```python
from build123d import *

# Parameters (mm, degrees)
SKETCH1_R           = 15.875
BOSS_EXTRUDE1_DEPTH = 50.8
SKETCH2_R           = 6.35
BOSS_EXTRUDE2_DEPTH = 6.35
SKETCH3_R           = 1.5875
BOSS_EXTRUDE3_DEPTH = 3.175
SKETCH4_R           = 3.175
BOSS_EXTRUDE4_DEPTH = 2.54
BOSS_EXTRUDE5_START = 19.05
SKETCH5_R           = 1.5875
BOSS_EXTRUDE5_DEPTH = 19.05
CUT_EXTRUDE1_DEPTH  = 6.35
SKETCH7_R           = 1.27
CUT_EXTRUDE2_DEPTH  = 8.89


with BuildPart() as part:
    # Sketch1 → Boss-Extrude1 (new body)
    with BuildSketch(Plane.XY):
        Circle(SKETCH1_R)
    extrude(amount=BOSS_EXTRUDE1_DEPTH)

    # Sketch2 → Boss-Extrude2 (add)
    with BuildSketch(Plane(origin=(0, 0, 0), x_dir=(-1, 0, 0), z_dir=(0, 0, -1))):
        with Locations(Location((0, 0, 0), (0, 0, 180))):
            Circle(SKETCH2_R)
    extrude(amount=BOSS_EXTRUDE2_DEPTH)

    # Sketch3 → Boss-Extrude3 (add)
    with BuildSketch(Plane(origin=(0, 0, -6.35), x_dir=(-1, 0, 0), z_dir=(0, 0, -1))):
        Circle(SKETCH3_R)
    extrude(amount=BOSS_EXTRUDE3_DEPTH)

    # Sketch4 → Boss-Extrude4 (add)
    with BuildSketch(Plane.XY.offset(50.8)):
        Circle(SKETCH4_R)
    extrude(amount=BOSS_EXTRUDE4_DEPTH)

    # Sketch5 → Boss-Extrude5 (add)
    with BuildSketch(Plane.XY.offset(53.34).offset(BOSS_EXTRUDE5_START)):
        with Locations(Location((0, 0, 0), (0, 0, 180))):
            Circle(SKETCH5_R)
    extrude(amount=-BOSS_EXTRUDE5_DEPTH)

    # Sketch6 → Cut-Extrude1 (cut)
    with BuildSketch(Plane.XY.offset(72.39)):
        with BuildLine():
            Line((-0.9525, 1.27), (0.9525, 1.27))
            ThreePointArc((0.9525, 1.27), (0, 1.5875), (-0.9525, 1.27))
        make_face()
    extrude(amount=-CUT_EXTRUDE1_DEPTH, mode=Mode.SUBTRACT)

    # Sketch7 → Cut-Extrude2 (cut)
    with BuildSketch(Plane.XY.offset(50.8)):
        with Locations((0, 9.525)):
            Circle(SKETCH7_R)
        with Locations((9.525, 0)):
            Circle(SKETCH7_R)
        with Locations((0, -9.525)):
            Circle(SKETCH7_R)
        with Locations((-9.525, 0)):
            Circle(SKETCH7_R)
    extrude(amount=-CUT_EXTRUDE2_DEPTH, mode=Mode.SUBTRACT)


solid = part.part
```
Can you work these out from the model? Positions are in its coordinate system, mm. A direction names the side the tool comes from. Give positions to 0.01 mm unless a question says otherwise; leave off trailing zeros. Write each loop counter-clockwise with the first axis right and the second up, starting at its lowest first coordinate (ties: lowest second). Pieces come first, ordered by that corner, then holes. Notation, with made-up numbers: (57.5, 61) - (80.5, 61) arc R19 cw to (80.5, 87) - close; hole circle Ø10 at (-1.75, 83.25). An arc over 180 degrees is marked (long way). Write item = value, one per line. Start each with the question number.
1. Thinking about a two-plate mould opening in X: for faces 6 (the face through (10, 0, 41.91)), 7 (the face through (1.3, 1.3, -6.35)), 8 (the face through (-0.69, -3.1, 52.05)), which applies, released by +X, released by -X, zero draft, split by the parting line, or undercut?
2. For pin 1 (2 mm diameter, centred on x = 9.525, y = 0, fed in from -Z); pin 2 (1 mm diameter, centred on x = 1.5, z = 28.5, fed in from -Y); pin 3 (5 mm diameter, centred on x = 11.5, y = 3.5, fed in from +Z), each with a flat end and sliding along its axis, tell me the tip position at first contact or that it passes through.
3. Imagine slicing it at C-C (z = 47). Please give me the cut outline in (x, y) (3 decimals).
4. Please list where these lines run through material, in increasing order: line 1 (Y direction, x = 0, z = 45.5) (3 decimals); line 2 (Z direction, x = -1, y = 13.5); line 3 (Y direction, x = 0, z = 16) (3 decimals).
5. Imagine slicing it at D-D (z = 2). Please give me the cut outline in (x, y) (3 decimals), and give its area (3 significant figures).
6. On a 3-axis mill with a long thin cutter (end or side, diameter ignored), from which of +Z, -Z, +X, -X, +Y, -Y can I reach the whole of each face in a straight line? I mean faces 1 (the face through (0, 0, -9.525)), 2 (the face through (0, 1.27, 69)), 3 (the face through (-0.165, -8.266, 46.417)), 4 (the face through (0, 0, 72.39)), 5 (the face through (7, 0, 0)). Say none if no direction works.
Worked answers:
q1.face_6 = undercut
q1.face_7 = zero draft
q1.face_8 = split by the parting line
q2.pin_1 = 0
q2.pin_2 = -15.84
q2.pin_3 = 50.8
q3.outline = circle Ø31.75 at (0, 0); hole circle Ø2.54 at (-9.525, 0); hole circle Ø2.54 at (0, -9.525); hole circle Ø2.54 at (0, 9.525); hole circle Ø2.54 at (9.525, 0)
q4.line_1 = -15.875 to -10.795, -8.255 to 8.255, 10.795 to 15.875
q4.line_2 = 0 to 50.8
q4.line_3 = -15.875 to 15.875
q5.outline = circle Ø31.75 at (0, 0)
q5.area = 792 mm2
q6.face_1 = -Z, +X, -X, +Y, -Y
q6.face_2 = +Z, +X, -X, +Y
q6.face_3 = +Z
q6.face_4 = +Z, +X, -X, +Y, -Y
q6.face_5 = -Z
